Autodesk Inventor part; units mm, degrees
ref_plane "YZ Plane" through (0, 0, 0) normal (1, 0, 0) x (0, 1, 0)
ref_plane "XZ Plane" through (0, 0, 0) normal (0, 1, 0) x (-1, 0, 0)
ref_plane "XY Plane" through (0, 0, 0) normal (0, 0, 1) x (1, 0, 0)
sketch "Sketch1" plane through (0, 0, 0) normal (0, 1, 0) x (-1, 0, 0)
  line L0 (34, 91) -> (34, 0)
  arc A0 (-34, 0) -> (34, 0) centre (0, 0) ccw
  line L1 (-34, 0) -> (-34, 80)
  line L2 (-34, 80) -> (4, 80)
  line L3 (4, 80) -> (4, 91)
  arc A1 (34, 91) -> (4, 91) centre (19, 91) ccw
  dimension "d0" = 34
  dimension "d1" = 15
  dimension "d2" = 91
  dimension "d3" = 80
extrude "Extrusion1" add sketch "Sketch1" along normal blind 40
sketch "Sketch2" plane through (0, 40, 0) normal (0, 1, 0) x (1, 0, 0)
  line L0 (-4, -80) -> (34, -80)
  arc A0 (34, 0) -> (-34, 0) centre (0, 0) ccw
  line L1 (-4, -80) -> (4, -80)
  line L2 (4, -80) -> (4, 0)
  line L3 (4, 0) -> (-4, 0)
  line L4 (-4, 0) -> (-4, -80)
  dimension "d6" = 8
extrude "Extrusion2" cut sketch "Sketch2" against normal through all
sketch "Sketch3" plane through (-4, 0, 91) normal (1, 0, 0) x (0, 0, -1)
  line L0 (0, 40) -> (91, 40)
  line L1 (11, 0) -> (11, 40)
  line L2 (-15, 0) -> (-15, 40)
  line L3 (11, 40) -> (-15, 40)
  line L4 (-15, 40) -> (-15, 12)
  line L5 (-15, 12) -> (11, 12)
  line L6 (11, 12) -> (11, 40)
  line L7 (0, 0) -> (-15, 0)
  point P0 (11, 12)
  dimension "d9" = 12
extrude "Extrusion3" cut sketch "Sketch3" against normal through all
sketch "Sketch4" plane through (0, 0, 0) normal (0, -1, 0) x (1, 0, 0)
  line L0 (4, 80) -> (4, 0)
  line L1 (4, 0) -> (-4, 0)
  line L2 (-4, 91) -> (-4, 0)
  arc A0 (-34, 0) -> (34, 0) centre (0, 0) ccw
  circle A1 centre (0, 0) radius 30
  point P0 (-4, 29.7321)
  point P1 (4, 29.7321)
  dimension "d12" = 60
extrude "Extrusion4" add sketch "Sketch4" along normal blind 30
chamfer "Chamfer1" distance 2 angle 45 1 edges at (-4, -30, -29.7321)
fillet "Fillet1" radius 4 2 edges at (-19, 40, 80) (19, 40, 80)
sketch "Sketch5" plane through (-4, 12, 91) normal (0, 1, 0) x (1, 0, 0)
  arc A0 (-30, 0) -> (0, 0) centre (-15, 0) ccw
  point P0 (4, 91)
hole "Hole1" at (-19, 12, 91) direction (0, -1, 0) diameter 14 end through all
sketch "Sketch6" plane through (0, -30, 0) normal (0, -1, 0) x (1, 0, 0)
  circle A0 centre (0, 0) radius 28
hole "Hole2" at (0, -30, 0) direction (0, 1, 0) diameter 50 end through all
sketch "Sketch7" plane through (34, 0, 80) normal (1, 0, 0) x (0, 0, -1)
  line L0 (80, 0) -> (80, 40)
  line L1 (4, 40) -> (80, 40)
  point P0 (20, 20)
  dimension "d33" = 60
  dimension "d34" = 20
hole "Hole3" at (34, 20, 60) direction (-1, 0, 0) diameter 12 end through all counterbore diameter 20 counterbore depth 10
properties part number "Part030. Notched attach" material "Steel, Cast"
Read the model definition and answer for the solid it produces. Units are mm, in the model's axes. A direction names the side the tool comes from. Coordinates: 2 decimals unless noted, no trailing zeros. Write each loop counter-clockwise with the first axis right and the second up, starting at its lowest first coordinate (ties: lowest second). Pieces come first, ordered by that corner, then holes. Notation, with made-up numbers: (-12.5, 70.25) -> (7.5, 70.25) arc R16 ccw to (7.5, 86.25) -> close; hole circle Ø6 at (88.25, 40). An arc over 180 degrees is marked (long way). Return JSON: item names as keys, results as strings.
(1) Which of the six approach directions +Z, -Z, +X, -X, +Y, -Y give full straight-line access (tool end or side, diameter ignored) to faces 1 (the flat face through (0, 0, 27)), 2 (the flat face through (24, 27, 60)), 3 (the flat face through (19, 18, 80))?
Answers below:
{"face 1": "+Z, +Y", "face 2": "+X", "face 3": "+Z, +X, +Y, -Y"}
(2) The part is cut by section D-D on z = 40. Give the vertices of the cut face in (x, y).
Answers below:
{"outline": "(-34, 0) -> (-4, 0) -> (-4, 40) -> (-34, 40) -> close; (4, 0) -> (34, 0) -> (34, 40) -> (4, 40) -> close"}
(3) Each of these flat-tipped pins is pushed along its axis until it touches: P1, Ø21, axis at x = -23.5, z = 88, coming from the +Y side; P2, Ø6, axis at x = -21.5, y = -17.5, coming from the +Z side; P3, Ø1.5, axis at x = 21.5, y = -20.5, coming from the -Z side; P4, Ø12.5, axis at x = -19, z = 91, coming from the -Y side (3 decimals). Where does it stop, or does it pass through?
Answers below:
{"P1": "y = 39.71", "P2": "z = 23.62", "P3": "z = -21.67", "P4": "through"}
(4) The part is cut by section B-B on z = 60. Give the vertices of the cut face in (x, y), then the cut area to 3 significant figures.
Answers below:
{"outline": "(-34, 0) -> (-4, 0) -> (-4, 14) -> (-34, 14) -> close; (-34, 26) -> (-4, 26) -> (-4, 40) -> (-34, 40) -> close; (4, 0) -> (34, 0) -> (34, 10) -> (24, 10) -> (24, 14) -> (4, 14) -> close; (4, 26) -> (24, 26) -> (24, 30) -> (34, 30) -> (34, 40) -> (4, 40) -> close", "area": "1,600 mm^2"}
(5) The part is cut by section A-A on x = 0. Give the vertices of the cut face in (y, z), then the cut area to 3 significant figures.
Answers below:
{"outline": "(-30, -28) -> (-28, -30) -> (0, -30) -> (0, -34) -> (40, -34) -> (40, -25) -> (-30, -25) -> close; (-30, 25) -> (0, 25) -> (0, 30) -> (-28, 30) -> (-30, 28) -> close", "area": "656 mm^2"}
(6) The part is cut by section C-C on y = 17. Give the vertices of the cut face in (x, z).
Answers below:
{"outline": "(-34, 0) arc R34 ccw to (34, 0) -> (34, 50.46) -> (24, 50.46) -> (24, 54.8) -> (4, 54.8) -> (4, 24.68) arc R25 cw (long way) to (-4, 24.68) -> (-4, 54.8) -> (-34, 54.8) -> close; (-34, 65.2) -> (-4, 65.2) -> (-4, 80) -> (-34, 80) -> close; (4, 65.2) -> (24, 65.2) -> (24, 69.54) -> (34, 69.54) -> (34, 80) -> (4, 80) -> close"}
(7) For a pull along Z with two mould halves and no side action, classify faces 4 (the flat face through (-19, 24, 80)), 5 (the cylindrical face through (-7.509, 5.49, -23.846)), 6 (the flat face through (-34, 20, 46)), 7 (the conical face through (-6.1, -29.87, 27.46)) as pulls with the +Z half, pulls with the -Z half, needs draft (parallel to the pull), parting line crosses it, or undercut.
Answers below:
{"face 4": "pulls with the +Z half", "face 5": "undercut", "face 6": "needs draft", "face 7": "parting line crosses it"}
(8) Consider line 1 along Z through (x, y) = (-19, 5.25); line 2 along X through (y, z) = (22, 40); line 3 along Y through (x, z) = (26.5, 21.5). Determine where each line is inside the solid, lowest interval first. Write a range as from..to.
Answers below:
{"line 1": "-28.2..-16.25, 16.25..84, 98..106", "line 2": "-34..-4, 4..34", "line 3": "0..40"}
